```python
from build123d import *

# Parameters (mm, degrees)
F1_DEPTH = 11
F2_R     = 2.85
F3_DEPTH = 25
F4_W     = 3
F4_H     = 7.1
F5_DEPTH = 10
F6_R     = 2
F7_DEPTH = 3


with BuildPart() as f1:
    # F0 (on Top) → F1 (new body)
    with BuildSketch(Plane.XY):
        with BuildLine():
            Line((-15.7, 1.7), (-15.7, 0))
            Line((-15.7, 0), (0, 0))
            Line((0, 0), (0, 12.6))
            Line((0, 12.6), (-15.7, 12.6))
            Line((-15.7, 12.6), (-15.7, 10.9))
            ThreePointArc((-15.7, 10.9), (-16.285786, 9.485786), (-17.7, 8.9))
            Line((-17.7, 8.9), (-26.7, 8.9))
            Line((-26.7, 8.9), (-26.7, 3.7))
            Line((-26.7, 3.7), (-17.7, 3.7))
            ThreePointArc((-17.7, 3.7), (-16.285786, 3.114214), (-15.7, 1.7))
        make_face()
        with BuildLine():
            ThreePointArc((-6, 4.15), (-6.146447, 3.796447), (-6.5, 3.65))
            Line((-6.5, 3.65), (-10.35, 3.65))
            ThreePointArc((-10.35, 3.65), (-13, 6.3), (-10.35, 8.95))
            Line((-10.35, 8.95), (-6.5, 8.95))
            ThreePointArc((-6.5, 8.95), (-6.146447, 8.803553), (-6, 8.45))
            Line((-6, 8.45), (-6, 4.15))
        make_face(mode=Mode.SUBTRACT)
    extrude(amount=F1_DEPTH)

    # F2 (on face) → F3 (cut)
    with BuildSketch(Plane.XZ.offset(-3.7)):
        with Locations((-20.550203, 5.55)):
            Circle(F2_R)
    extrude(amount=-F3_DEPTH, mode=Mode.SUBTRACT)

    # F4 (on face) → F5 (cut)
    with BuildSketch(Plane(origin=(0, 0, 0), x_dir=(1, 0, 0), z_dir=(0, 0, -1))):
        with Locations((-4.5, -6.3)):
            Rectangle(F4_W, F4_H)
    extrude(amount=-F5_DEPTH, mode=Mode.SUBTRACT)

    # F6 (on face) → F7 (cut, through all)
    with BuildSketch(Plane.YZ):
        with Locations((6.3, 5.5)):
            Circle(F6_R)
    extrude(amount=-F7_DEPTH, mode=Mode.SUBTRACT)


solid = f1.part
```
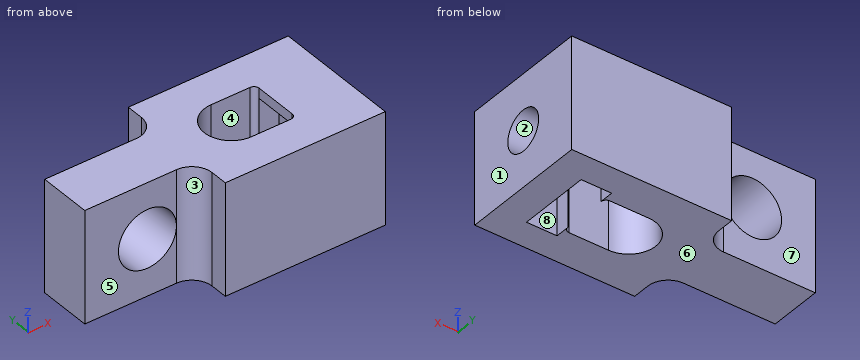
Can you work these out from the model? Positions are in its coordinate system, mm. Face numbers are marked on the shaded views. A direction names the side the tool comes from. Round coordinates to 2 decimals unless told otherwise and drop trailing zeros. Loops run counter-clockwise (first coordinate to the right, second up) from the corner with the lowest first, then second, coordinate; pieces in that order, holes last. Notation, with made-up numbers: M 18.5,77.25 L 48.5,77.25 A16 cw 48.5,82.25 Z; hole C 40.5,51 d1. An arc over 180 degrees is marked long. Answer in a Markdown table with one row per item.
1. If we section it at D-D, the plane z = 1.5: Please give me the cut outline in (x, y), plus the area to 3 significant figures.
Established:
| item | result |
|---|---|
| outline | M -26.7,3.7 L -17.7,3.7 A2 cw -15.7,1.7 L -15.7,0 L 0,0 L 0,12.6 L -15.7,12.6 L -15.7,10.9 A2 cw -17.7,8.9 L -26.7,8.9 Z; hole M -10.35,3.65 L -6.5,3.65 A0.5 ccw -6,4.15 L -6,2.75 L -3,2.75 L -3,9.85 L -6,9.85 L -6,8.45 A0.5 ccw -6.5,8.95 L -10.35,8.95 A2.65 ccw Z |
| area | 201 mm² |
2. If we section it at C-C, the plane z = 6.5: Please give me the cut outline in (x, y).
Established:
| item | result |
|---|---|
| outline | M -26.7,3.7 L -23.24,3.7 L -23.24,8.9 L -26.7,8.9 Z; M -17.86,3.7 L -17.7,3.7 A2 cw -15.7,1.7 L -15.7,0 L 0,0 L 0,4.57 L -3,4.57 L -3,2.75 L -6,2.75 L -6,4.15 A0.5 cw -6.5,3.65 L -10.35,3.65 A2.65 cw -10.35,8.95 L -6.5,8.95 A0.5 cw -6,8.45 L -6,9.85 L -3,9.85 L -3,8.03 L 0,8.03 L 0,12.6 L -15.7,12.6 L -15.7,10.9 A2 cw -17.7,8.9 L -17.86,8.9 Z |
3. If we section it at B-B, the plane x = -8.25: Please give me the cut outline in (y, z).
Established:
| item | result |
|---|---|
| outline | M 0,0 L 3.65,0 L 3.65,11 L 0,11 Z; M 8.95,0 L 12.6,0 L 12.6,11 L 8.95,11 Z |
4. Thinking about a two-plate mould opening in Y: for the marked faces 1, 2 and 3, which applies, pulls with the +Y half, pulls with the -Y half, needs draft (parallel to the pull), parting line crosses it, or undercut?
Established:
| item | result |
|---|---|
| face 1 | needs draft |
| face 2 | undercut |
| face 3 | pulls with the -Y half |
5. I'm going to push flat-ended pins straight in: pin 1 Ø5 at (y, z) = (6.5, 8.5) entering from +X; pin 2 Ø0.8 at (y, z) = (1, 3) entering from -X; pin 3 Ø2.5 at (x, z) = (-24.5, 5.5) entering from -Y; pin 4 Ø2.5 at (x, z) = (-20, 3) entering from +Y. Where does each tip first touch, or does it pass through?
Established:
| item | result |
|---|---|
| pin 1 | x = 0 |
| pin 2 | x = -15.7 |
| pin 3 | y = 3.7 |
| pin 4 | y = 8.9 |
6. On a 3-axis mill with a long thin cutter (end or side, diameter ignored), from which of +Z, -Z, +X, -X, +Y, -Y can I reach the whole of each face in a straight line? I mean the marked faces 4, 5, 6, 7 and 8. Say none if no direction works.
Established:
| item | result |
|---|---|
| face 4 | +Z, -Z |
| face 5 | +Z, -Z, -X, -Y |
| face 6 | -Z, +X, -X, +Y, -Y |
| face 7 | +Z, -Z, -X, +Y |
| face 8 | -Z |
7. Please list where these lines run through material, in increasing order: line 1 (Y direction, x = -9.25, z = 2); line 2 (Y direction, x = -4.5, z = 9.5); line 3 (Z direction, x = -1.8, y = 6.3). Write a range as from..to.
Established:
| item | result |
|---|---|
| line 1 | 0..3.65, 8.95..12.6 |
| line 2 | 0..2.75, 9.85..12.6 |
| line 3 | 0..3.5, 7.5..11 |
8. If we section it at A-A, the plane y = 6.3: Please give me the cut outline in (x, z).
Established:
| item | result |
|---|---|
| outline | M -26.7,0 L -13,0 L -13,11 L -26.7,11 Z; M -6,10 L -3,10 L -3,7.5 L 0,7.5 L 0,11 L -6,11 Z; M -3,0 L 0,0 L 0,3.5 L -3,3.5 Z; hole C -20.55,5.55 d5.7 |
